CAD build for the part. Positions are in the model's coordinates, mm. Face numbers are marked on the shaded views. A direction names the side the tool comes from. Give positions to 0.01 mm unless a question says otherwise; leave off trailing zeros. Loops run counter-clockwise (first coordinate to the right, second up) from the corner with the lowest first, then second, coordinate; pieces in that order, holes last. Notation, with made-up numbers: (-19.5, -33.75) - (19.5, -33.75) arc R31 cw to (19.5, 4.25) - close; hole circle Ø3 at (78.5, -2). An arc over 180 degrees is marked (long way). Return JSON: item names as keys, results as strings.
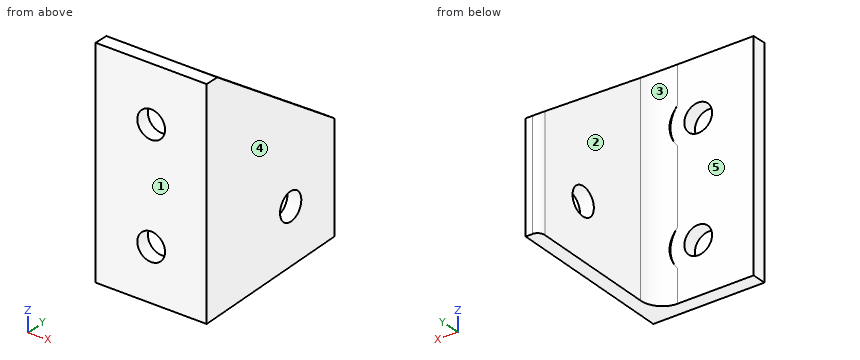
from build123d import *

# Parameters (mm, degrees)
BOSS_EXTRUDE1_DEPTH = 25.4
SKETCH3_R           = 3.175
SKETCH3_W           = 12.7
SKETCH3_H           = 50.8
CUT_EXTRUDE1_DEPTH  = 50.595085442
SKETCH12_OUTSIDE_W  = 66.478
SKETCH12_OUTSIDE_H  = 53.778
CUT_EXTRUDE2_DEPTH  = 41.659838908
SKETCH13_R          = 3.175
CUT_EXTRUDE3_DEPTH  = 41.659838908
SKETCH14_R          = 6.35
CUT_EXTRUDE4_DEPTH  = 2.54


with BuildPart() as part:
    # Sketch2 → Boss-Extrude1 (new, symmetric)
    with BuildSketch(Plane.XY):
        with BuildLine():
            Line((-19.05, -19.05), (19.05, -19.05))
            Line((19.05, -19.05), (19.05, 19.05))
            Line((19.05, 19.05), (17.4625, 19.05))
            ThreePointArc((17.4625, 19.05), (16.339967985, 18.585032015), (15.875, 17.4625))
            Line((15.875, 17.4625), (15.875, -11.0998))
            ThreePointArc((15.875, -11.0998), (14.476376302, -14.476376302), (11.0998, -15.875))
            Line((11.0998, -15.875), (-17.4625, -15.875))
            ThreePointArc((-17.4625, -15.875), (-18.585032015, -16.339967985), (-19.05, -17.4625))
            Line((-19.05, -17.4625), (-19.05, -19.05))
        make_face()
    extrude(amount=BOSS_EXTRUDE1_DEPTH, both=True)

    # Sketch3 → Cut-Extrude1 (cut, through all)
    with BuildSketch(Plane.XZ.offset(19.05)):
        with Locations((6.35, 12.7)):
            Circle(SKETCH3_R)
        with Locations((6.35, -12.7)):
            Circle(SKETCH3_R)
        with Locations((-12.7, 0)):
            Rectangle(SKETCH3_W, SKETCH3_H)
    extrude(amount=-CUT_EXTRUDE1_DEPTH, mode=Mode.SUBTRACT)

    # Sketch12 outside → Cut-Extrude2 (cut, through all)
    with BuildSketch(Plane(origin=(19.05, 0, 0), x_dir=(0, 0, -1), z_dir=(1, 0, 0))):
        Rectangle(SKETCH12_OUTSIDE_W, SKETCH12_OUTSIDE_H)
        Polygon((23.087203004, 19.05), (24.449518438, -19.05), (-25.4, -19.05), (-25.4, -15.875), (-1.48415665, 19.05), align=None, mode=Mode.SUBTRACT)
    extrude(amount=-CUT_EXTRUDE2_DEPTH, mode=Mode.SUBTRACT)

    # Sketch13 → Cut-Extrude3 (cut, through all)
    with BuildSketch(Plane(origin=(19.05, 0, 0), x_dir=(0, 0, -1), z_dir=(1, 0, 0))):
        with Locations(Location((11.088634042, 6.021904729, 0), (0, 0, 90))):
            Circle(SKETCH13_R)
    extrude(amount=-CUT_EXTRUDE3_DEPTH, mode=Mode.SUBTRACT)

    # Sketch14 → Cut-Extrude4 (cut)
    with BuildSketch(Plane(origin=(0, -15.875, 0), x_dir=(1, 0, 0), z_dir=(0, 1, 0))):
        with Locations((6.35, -12.7)):
            Circle(SKETCH14_R)
        with Locations((6.35, 12.7)):
            Circle(SKETCH14_R)
    extrude(amount=CUT_EXTRUDE4_DEPTH, mode=Mode.SUBTRACT)


solid = part.part
1. Drop flat-ended pins along their axis: P1, Ø5, axis at x = -3, z = 6.5, coming from the +Y side (3 decimals); P2, Ø12, axis at y = 8, z = 15, coming from the -X side (3 decimals); P3, Ø5.5, axis at y = 6.02, z = -11.09, coming from the +X side. Give the stop position or say it passes through.
Values follow:
{"P1": "stops at y = -15.875", "P2": "stops at x = 15.875", "P3": "passes through"}
2. Cut at B-B, the plane z = -12.7. Give the number of separate pieces and of enclosed holes in the cut face, plus the area to 3 significant figures.
Values follow:
{"separate pieces": "3", "enclosed holes": "0", "area": "158 mm²"}
3. Cut at A-A, the plane x = 6.35. Write the cut outline in (y, z) (3 decimals).
Values follow:
{"outline": "(-19.05, -24.45) - (-15.875, -24.336) - (-15.875, -15.875) - (-19.05, -15.875) - close; (-19.05, -9.525) - (-15.875, -9.525) - (-15.875, 9.525) - (-19.05, 9.525) - close; (-19.05, 15.875) - (-15.875, 15.875) - (-15.875, 25.4) - (-19.05, 25.4) - close"}
4. Which spindle directions (+Z, -Z, +X, -X, +Y, -Y) get a long thin tool onto all of the face, cutting with end or side? Do the marked faces 1 and 2. Say none if no direction does.
Values follow:
{"face 1": "+Z, -Z, +X, -X, -Y", "face 2": "+Z, -Z, -X, +Y"}
5. Cut at C-C, the plane z = 12.7. Write the cut outline in (x, y) (3 decimals).
Values follow:
{"outline": "(-6.35, -19.05) - (3.175, -19.05) - (3.175, -15.875) - (-6.35, -15.875) - close; (9.525, -19.05) - (19.05, -19.05) - (19.05, 2.671) - (15.875, 2.671) - (15.875, -11.1) arc R4.775 cw to (12.7, -15.599) - (12.7, -15.875) - (9.525, -15.875) - close"}
6. Pull direction X, two halves, no side cores. Call the marked faces 3, 4 and 5: +X half, -X half, draft (parallel to the pull), parting line (faces both ways), or undercut.
Values follow:
{"face 3": "-X half", "face 4": "+X half", "face 5": "draft"}
7. Drill centre lines: probe 1 along Z at (x, y) = (6.35, -17.2) (3 decimals); probe 2 along X at (y, z) = (2.5, -4.5) (3 decimals); probe 3 along Y at (x, z) = (-0.75, 11.5) (3 decimals). Where is each one in solid material? Low to high.
Values follow:
{"probe 1": "z = -24.383 to -15.875, -9.525 to 9.525, 15.875 to 25.4", "probe 2": "x = 15.875 to 19.05", "probe 3": "y = -19.05 to -15.875"}
